Geometry: final body of the model. Coordinates: model frame, mm. Face numbers are marked on the shaded views. A direction names the side the tool comes from. Round coordinates to 2 decimals unless told otherwise and drop trailing zeros. Loops run counter-clockwise (first coordinate to the right, second up) from the corner with the lowest first, then second, coordinate; pieces in that order, holes last. Notation, with made-up numbers: (-8, 9.25) - (40, 9.25) arc R18 ccw to (40, 43.25) - close; hole circle Ø2 at (88, 54.5). An arc over 180 degrees is marked (long way). Return JSON: item names as keys, results as strings. Group by question number.
1. Section A-A on z = 39. Return loops of the section in (x, y), and give its area (3 significant figures).
2. Section C-C on x = 87. Return loops of the section in (y, z), and give its area (3 significant figures).
3. Draft query along Y for the marked faces 1, 2, 3 and 4. Return one class per face: +Y half, -Y half, draft (parallel to the pull), parting line (faces both ways), or undercut.
4. Material intervals for probe 1 along Y at (x, z) = (100, 10.5); probe 2 along Z at (x, y) = (32, 21); probe 3 along Y at (x, z) = (50, 33), sorted ascending.
5. Set-up query: the marked faces 5, 6, 7, 8 and 9. Return all of +Z, -Z, +X, -X, +Y, -Y with unobstructed straight access to the full face (end or side cutting, diameter ignored); none if empty.
6. Section D-D on y = 29. Return loops of the section in (x, z), and give its area (3 significant figures).
7. Section B-B on y = 21. Return loops of the section in (x, z).
8. First-contact query: pin 1 Ø1.5 at (y, z) = (57.5, 41) entering from +X; pin 2 Ø5 at (x, y) = (53, 42.5) entering from +Z; pin 3 Ø5 at (y, z) = (42, 36.5) entering from -X. Flat tips, straight axial feed; report the tip coordinate or a pass-through.
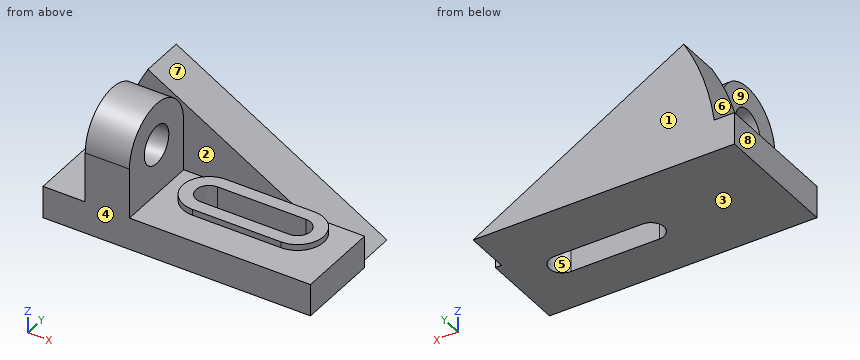
from build123d import *

# Parameters (mm, degrees)
F1_DEPTH  = 42
F2_W      = 121
F2_H      = 22
F3_ANGLE  = 30
F5_DEPTH  = 22
F8_DEPTH  = 3
F9_DEPTH  = 25
F6_R      = 9.5
F10_DEPTH = 25
F11_W     = 10.0625162845
F11_H     = 22
F12_DEPTH = 16


with BuildPart() as f1:
    # F0 (on Front) → F1 (new body)
    with BuildSketch(Plane.XZ):
        Polygon((0, 16), (0, 0), (133, 0), (133, 16), (43, 16), (43, 41), (21, 41), (21, 16), align=None)
    extrude(amount=-F1_DEPTH)

    # F2 (on Top) → F3 (revolve)
    with BuildSketch(Plane.XY):
        with Locations((69.5, 53)):
            Rectangle(F2_W, F2_H)
    revolve(axis=Axis((130, 53, 0), (0, 1, 0)), revolution_arc=F3_ANGLE)

    # F4 (on face) → F5 (join)
    with BuildSketch(Plane.YZ.offset(43)):
        with BuildLine():
            Line((0, 41), (42, 41))
            ThreePointArc((42, 41), (21, 62), (0, 41))
        make_face()
    extrude(amount=-F5_DEPTH)

    # F7 (on face) → F8 (join)
    with BuildSketch(Plane.XY.offset(16)):
        with BuildLine():
            Line((102.2871870789, 42), (64, 42))
            ThreePointArc((64, 42), (51, 29), (64, 16))
            Line((64, 16), (108, 16))
            ThreePointArc((108, 16), (121, 29), (108, 42))
            Line((108, 42), (102.2871870789, 42))
        make_face()
        with BuildLine():
            ThreePointArc((64, 22.5), (57.5, 29), (64, 35.5))
            Line((64, 35.5), (108, 35.5))
            ThreePointArc((108, 35.5), (114.5, 29), (108, 22.5))
            Line((108, 22.5), (64, 22.5))
        make_face(mode=Mode.SUBTRACT)
    extrude(amount=F8_DEPTH)

    # F9 (cut): a face of the model
    f9_faces = [f1.faces().sort_by_distance(p)[0] for p in [
        (86, 29, 16),
    ]]
    extrude(f9_faces, amount=-F9_DEPTH, mode=Mode.SUBTRACT)

    # F6 (on face) → F10 (cut)
    with BuildSketch(Plane.YZ.offset(43)):
        with Locations((21, 41)):
            Circle(F6_R)
    extrude(amount=-F10_DEPTH, mode=Mode.SUBTRACT)

    # F11 (on face) → F12 (join)
    with BuildSketch(Plane.XY.offset(16)):
        with Locations((5.0312581423, 53)):
            Rectangle(F11_W, F11_H)
    extrude(amount=-F12_DEPTH)


solid = f1.part
Taken from the geometry:
{
 "1": {"outline": "(15.46, 42) - (21, 42) - (21, 30.29) - (43, 30.29) - (43, 42) - (62.45, 42) - (62.45, 64) - (15.46, 64) - close; (21, 0) - (43, 0) - (43, 11.71) - (21, 11.71) - close", "area": "1,550 mm2"},
 "2": {"outline": "(0, 0) - (22.5, 0) - (22.5, 19) - (16, 19) - (16, 16) - (0, 16) - close; (35.5, 0) - (64, 0) - (64, 24.83) - (42, 24.83) - (42, 19) - (35.5, 19) - close", "area": "1,050 mm2"},
 "3": {"face 1": "+Y half", "face 2": "undercut", "face 3": "draft", "face 4": "-Y half"},
 "4": {"probe 1": "0 to 22.5, 35.5 to 64", "probe 2": "0 to 31.5, 50.5 to 62", "probe 3": "42 to 64"},
 "5": {"face 5": "+Z, -Z", "face 6": "+Z, -X, +Y", "face 7": "+Z, +X, +Y", "face 8": "+Z, -Z, -X, +Y, -Y", "face 9": "+Z, -X, -Y"},
 "6": {"outline": "(0, 0) - (57.5, 0) - (57.5, 19) - (51, 19) - (51, 16) - (43, 16) - (43, 35.88) - (21, 35.88) - (21, 16) - (0, 16) - close; (21, 46.12) - (43, 46.12) - (43, 60.42) - (21, 60.42) - close; (114.5, 0) - (133, 0) - (133, 16) - (121, 16) - (121, 19) - (114.5, 19) - close", "area": "2,010 mm2"},
 "7": {"outline": "(0, 0) - (133, 0) - (133, 16) - (118.25, 16) - (118.25, 19) - (53.75, 19) - (53.75, 16) - (43, 16) - (43, 31.5) - (21, 31.5) - (21, 16) - (0, 16) - close; (21, 50.5) - (43, 50.5) - (43, 62) - (21, 62) - close"},
 "8": {"pin 1": "x = 60.28", "pin 2": "z = 45.9", "pin 3": "x = 13.88"}
}
